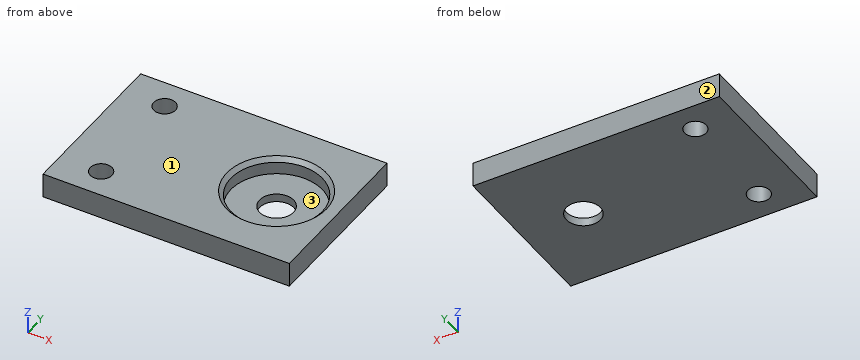
```python
from build123d import *

# Parameters (mm, degrees)
F0_W     = 40
F0_H     = 40
F0_R     = 11.15
F0_W_2   = 20
F0_R_2   = 2.65
F1_DEPTH = 6
F0_R_3   = 4.151826
F2_DEPTH = 2
F3_SIZE  = 1


with BuildPart() as f1:
    # F0 (on Top) → F1 (new body)
    with BuildSketch(Plane.XY):
        with Locations((-51.926523, 22.418201)):
            Rectangle(F0_W, F0_H)
        with Locations((-46.926523, 22.418201)):
            Circle(F0_R, mode=Mode.SUBTRACT)
        with Locations((-81.926523, 22.418201)):
            Rectangle(F0_W_2, F0_H)
        with Locations((-81.926523, 9.418201)):
            Circle(F0_R_2, mode=Mode.SUBTRACT)
        with Locations((-81.926523, 35.418201)):
            Circle(F0_R_2, mode=Mode.SUBTRACT)
    extrude(amount=F1_DEPTH)

    # F0 (on Top) → F2 (join)
    with BuildSketch(Plane.XY):
        with Locations((-46.926523, 22.418201)):
            Circle(F0_R)
        with Locations((-46.926523, 22.418201)):
            Circle(F0_R_3, mode=Mode.SUBTRACT)
    extrude(amount=F2_DEPTH)

    # F3
    f3_edges = [f1.edges().sort_by_distance(p)[0] for p in [
        (-58.076523, 22.418201, 6),
    ]]
    chamfer(f3_edges, length=F3_SIZE)


solid = f1.part
```
The listing builds one solid part. Answer for the finished solid, in the listing's coordinates (mm). Face numbers are marked on the shaded views. Give positions to 0.01 mm unless a question says otherwise; leave off trailing zeros. Write each loop counter-clockwise with the first axis right and the second up, starting at its lowest first coordinate (ties: lowest second). Pieces come first, ordered by that corner, then holes. Notation, with made-up numbers: (9.25, -11.5) - (36.25, -11.5) arc R30 cw to (36.25, 10.5) - close; hole circle Ø6 at (14, -26.5). An arc over 180 degrees is marked (long way). Use one line per item in the form item = value. Start each with the question number.
1) Find section A-A on z = 0.6. Determine the outline of the cut face in (x, y).
2) The mould has two halves that part along Y. Classify the marked faces 1, 2 and 3: pulls with the +Y half, pulls with the -Y half, needs draft (parallel to the pull), parting line crosses it, or undercut.
3) Flat-ended cylindrical pins translate along their axes: pin 1 Ø4 at (x, y) = (-39.5, 20.5) entering from +Z; pin 2 Ø3 at (x, y) = (-81.93, 9.42) entering from +Z. Find the tip coordinate at first contact, or state that the pin passes through.
4) Consider line 1 along X through (y, z) = (9.5, 2.7); line 2 along Z through (x, y) = (-42.5, 28.5); line 3 along Y through (x, z) = (-41.5, 2.9). Determine where each line is inside the solid, lowest interval first. Write a range as from..to.
Geometry results:
q1.outline = (-91.93, 2.42) - (-31.93, 2.42) - (-31.93, 42.42) - (-91.93, 42.42) - close; hole circle Ø5.3 at (-81.93, 9.42); hole circle Ø5.3 at (-81.93, 35.42); hole circle Ø8.3 at (-46.93, 22.42)
q2.face_1 = needs draft
q2.face_2 = pulls with the +Y half
q2.face_3 = undercut
q3.pin_1 = 2
q3.pin_2 = through
q4.line_1 = -91.93..-84.58, -79.28..-31.93
q4.line_2 = 0..2
q4.line_3 = 2.42..12.68, 32.16..42.42
